Input: part model. Units: mm. Frame: model coordinates. Face numbers are marked on the shaded views. A direction names the side the tool comes from. Round coordinates to 2 decimals unless told otherwise and drop trailing zeros. Order: outer loops, then holes, each group sorted by start corner. A loop starts at its lowest first (then second) coordinate and runs counter-clockwise, first axis right, second up.
Item 1: Cut plane A-A on z = 2. Output: boundary loops of the cut face in (x, y).
Item 2: Cut plane D-D on x = -23. Output: boundary loops of the cut face in (y, z), then the cut area to 3 significant figures.
Item 3: Line query: L1, parallel to X at y = -2.65, z = 4; L2, parallel to Y at x = -20, z = 1.25; L3, parallel to Y at x = 9.5, z = 4.5. Output: solid intervals per line, ascending.
Item 4: Cut plane B-B on y = -1. Output: boundary loops of the cut face in (x, z).
Item 5: Cut plane C-C on x = 4. Output: boundary loops of the cut face in (y, z), then the cut area to 3 significant figures.
Item 6: First-contact query: pin 1 (2 mm diameter, centred on x = -11, z = 2.5, fed in from +Y); pin 2 (2 mm diameter, centred on x = 8.64, z = 4, fed in from -Y). Flat tips, straight axial feed; report the tip coordinate or a pass-through.
Item 7: Reachability of the marked faces 1 and 2 from +Z, -Z, +X, -X, +Y, -Y: full face, straight path, thin tool, end or side. Return the list, or none.
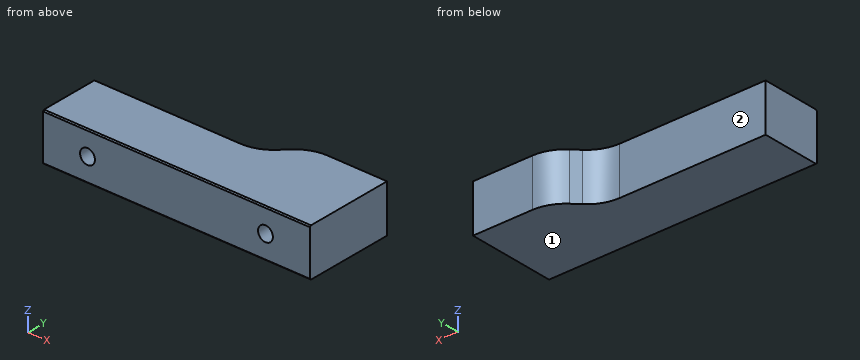
```python
from build123d import *

# Parameters (mm, degrees)
BOSS_EXTRUDE1_DEPTH   = 8
FILLET1_R             = 6.5
CHAMFER1_SIZE         = 0.2
M3_TAPPED_HOLE1_D     = 2.5
M3_TAPPED_HOLE1_DEPTH = 6
M3_TAPPED_HOLE1_TIP   = 0.751075774


with BuildPart() as part:
    # Sketch1 → Boss-Extrude1 (new body)
    with BuildSketch(Plane.XY):
        Polygon((-1.56097561, 4.365853659), (3.43902439, 9.365853659), (16.13902439, 9.365853659), (16.13902439, -5.634146341), (-28.86097561, -5.634146341), (-28.86097561, 4.365853659), align=None)
    extrude(amount=BOSS_EXTRUDE1_DEPTH)

    # Fillet1
    fillet1_edges = [part.edges().sort_by_distance(p)[0] for p in [
        (-1.56097561, 4.365853659, 4),
        (3.43902439, 9.365853659, 4),
    ]]
    fillet(fillet1_edges, radius=FILLET1_R)

    # Chamfer1
    chamfer1_edges = [part.edges().sort_by_distance(p)[0] for p in [
        (-6.36097561, -5.634146341, 8),
        (-6.36097561, -5.634146341, 0),
    ]]
    chamfer(chamfer1_edges, length=CHAMFER1_SIZE)

    # M3 Tapped Hole1
    with Locations(Plane(origin=(0, -5.634146341, 0), x_dir=(-1, 0, 0), z_dir=(0, -1, 0))):
        with Locations((21.36097561, -4), (-8.63902439, -4)):
            Hole(M3_TAPPED_HOLE1_D / 2, depth=M3_TAPPED_HOLE1_DEPTH)
            with Locations((0, 0, -(M3_TAPPED_HOLE1_DEPTH + M3_TAPPED_HOLE1_TIP / 2))):  # 118° drill point
                Cone(0, M3_TAPPED_HOLE1_D / 2, M3_TAPPED_HOLE1_TIP, mode=Mode.SUBTRACT)


solid = part.part
```
From the geometry:
1. outline: (-28.86, -5.63) - (16.14, -5.63) - (16.14, 9.37) - (6.13, 9.37) arc R6.5 ccw to (1.54, 7.46) - (0.34, 6.27) arc R6.5 cw to (-4.25, 4.37) - (-28.86, 4.37) - close
2. outline: (-5.63, 0.2) - (-5.43, 0) - (4.37, 0) - (4.37, 8) - (-5.43, 8) - (-5.63, 7.8) - close
2. area: 80.0 mm2
3. L1: x = -28.86 to -22.61, -20.11 to 7.39, 9.89 to 16.14
3. L2: y = -5.63 to 4.37
3. L3: y = 0.52 to 9.37
4. outline: (-28.86, 0) - (16.14, 0) - (16.14, 8) - (-28.86, 8) - close; hole circle Ø2.5 at (-21.36, 4); hole circle Ø2.5 at (8.64, 4)
5. outline: (-5.63, 0.2) - (-5.43, 0) - (9.01, 0) - (9.01, 8) - (-5.43, 8) - (-5.63, 7.8) - close
5. area: 117 mm2
6. pin 1: stops at y = 4.37
6. pin 2: stops at y = 0.52
7. face 1: -Z, +X, -X, +Y, -Y
7. face 2: +Z, -Z, -X, +Y
